```python
from build123d import *

# Parameters (mm, degrees)
SKETCH1_W                = 40.5
SKETCH1_H                = 20
BOSS_EXTRUDE1_DEPTH      = 36.1
SKETCH2_R                = 2.5
BOSS_EXTRUDE2_DEPTH      = 8
BOSS_EXTRUDE3_DEPTH      = 7.5
BOSS_EXTRUDE3_DEPTH_BACK = 48
SKETCH3_W                = 20
SKETCH3_H                = 2
SKETCH4_R                = 2
CUT_EXTRUDE1_DEPTH       = 7.5


with BuildPart() as part:
    # Sketch1 → Boss-Extrude1 (new body)
    with BuildSketch(Plane(origin=(0, 0, 0), x_dir=(1, 0, 0), z_dir=(0, 1, 0))):
        with Locations((3.506737992, 0.753901676)):
            Rectangle(SKETCH1_W, SKETCH1_H)
    extrude(amount=BOSS_EXTRUDE1_DEPTH)

    # Sketch2 → Boss-Extrude2 (add)
    with BuildSketch(Plane(origin=(0, 36.1, 0), x_dir=(1, 0, 0), z_dir=(0, 1, 0))):
        with Locations(Location((12.506737992, 0.753901676, 0), (0, 0, 270))):
            Circle(SKETCH2_R)
    extrude(amount=BOSS_EXTRUDE2_DEPTH)

    # Sketch3 → Boss-Extrude3 (add, two sides: drawn at the far end of the back side and taken through both)
    with BuildSketch(Plane.ZY.offset(16.743262008).offset(-BOSS_EXTRUDE3_DEPTH_BACK)):
        with Locations((-0.753901676, 27.6)):
            Rectangle(SKETCH3_W, SKETCH3_H)
    extrude(amount=BOSS_EXTRUDE3_DEPTH + BOSS_EXTRUDE3_DEPTH_BACK)

    # Sketch4 → Cut-Extrude1 (cut)
    with BuildSketch(Plane(origin=(0, 28.6, 0), x_dir=(1, 0, 0), z_dir=(0, 1, 0))):
        with Locations(Location((-20.493262008, 5.753901676, 0), (0, 0, 270))):
            Circle(SKETCH4_R)
        with Locations(Location((27.506737992, 5.753901676, 0), (0, 0, 270))):
            Circle(SKETCH4_R)
        with Locations(Location((-20.493262008, -4.246098324, 0), (0, 0, 270))):
            Circle(SKETCH4_R)
        with Locations(Location((27.506737992, -4.246098324, 0), (0, 0, 270))):
            Circle(SKETCH4_R)
    extrude(amount=-CUT_EXTRUDE1_DEPTH, mode=Mode.SUBTRACT)


solid = part.part
```
Geometry check sheet. Reference: the model listing, model coordinates, mm. A direction names the side the tool comes from. Coordinates: 2 decimals unless noted, no trailing zeros. Write each loop counter-clockwise with the first axis right and the second up, starting at its lowest first coordinate (ties: lowest second). Pieces come first, ordered by that corner, then holes. Notation, with made-up numbers: M 21.25,89.5 L 58.25,89.5 A20 ccw 58.25,127.5 Z; hole C -21.75,71.25 d9. An arc over 180 degrees is marked long. Use one line per item in the form item = value. Start each with the question number.
1) Section check A-A on z = 5.5. Enter the section's corners in (x, y).
2) Thickness scan on probe 1 along Y at (x, z) = (2, -4.25); probe 2 along X at (y, z) = (12.5, -8.5); probe 3 along Y at (x, z) = (24, 1.25). Record the ranges inside material, lowest first. Write a range as from..to.
3) Go/stop test with flat-tipped pins: pin 1 Ø8 at (x, z) = (-4, -4) entering from +Y; pin 2 Ø4 at (x, z) = (-21, 2) entering from -Y; pin 3 Ø3 at (x, z) = (-20.49, 4.25) entering from -Y; pin 4 Ø5 at (x, z) = (27.51, -5.75) entering from +Y. Record where each tip stops, or that it passes through.
4) Section check B-B on x = -19.5. Enter the section's corners in (y, z), and give its area (3 significant figures).
5) Release check for a two-part mould opening along Z. For faces 1 (the cylindrical face through (10.066, 40.044, -1.296)), 2 (the flat face through (28, 28.6, -1)), 3 (the cylindrical face through (27.595, 27.614, 2.248)) record: pulls with the +Z half, pulls with the -Z half, needs draft (parallel to the pull), parting line crosses it, or undercut.
6) Section check D-D on y = 15.5. Enter the section's corners in (x, z).
7) Set-up check for faces 4 (the flat face through (28, 26.6, -1)), 5 (the flat face through (-16.743, 13, -1)), 6 (the flat face through (3, 0, -1)), 7 (the flat face through (23.757, 32, -1)), 8 (the flat face through (-20, 28.6, -1)): record each of +Z, -Z, +X, -X, +Y, -Y from which the full face is reachable in a straight line by a thin tool's end or side.
8) Section check C-C on z = -9. Enter the section's corners in (x, y).
Responses:
q1.outline = M -24.24,26.6 L -22.05,26.6 L -22.05,28.6 L -24.24,28.6 Z; M -18.94,26.6 L -16.74,26.6 L -16.74,0 L 23.76,0 L 23.76,26.6 L 25.95,26.6 L 25.95,28.6 L 23.76,28.6 L 23.76,36.1 L -16.74,36.1 L -16.74,28.6 L -18.94,28.6 Z; M 29.06,26.6 L 31.26,26.6 L 31.26,28.6 L 29.06,28.6 Z
q2.probe_1 = 0..36.1
q2.probe_2 = -16.74..23.76
q2.probe_3 = 26.6..28.6
q3.pin_1 = 36.1
q3.pin_2 = 26.6
q3.pin_3 = through
q3.pin_4 = 28.6
q4.outline = M 26.6,-10.75 L 28.6,-10.75 L 28.6,-7.49 L 26.6,-7.49 Z; M 26.6,-4.02 L 28.6,-4.02 L 28.6,2.51 L 26.6,2.51 Z; M 26.6,5.98 L 28.6,5.98 L 28.6,9.25 L 26.6,9.25 Z
q4.area = 26.1 mm2
q5.face_1 = parting line crosses it
q5.face_2 = needs draft
q5.face_3 = undercut
q6.outline = M -16.74,-10.75 L 23.76,-10.75 L 23.76,9.25 L -16.74,9.25 Z
q7.face_4 = +Z, -Z, +X, -Y
q7.face_5 = +Z, -Z, -X, -Y
q7.face_6 = +Z, -Z, +X, -X, -Y
q7.face_7 = +Z, -Z, +X, +Y
q7.face_8 = +Z, -Z, -X, +Y
q8.outline = M -24.24,26.6 L -16.74,26.6 L -16.74,0 L 23.76,0 L 23.76,26.6 L 31.26,26.6 L 31.26,28.6 L 23.76,28.6 L 23.76,36.1 L -16.74,36.1 L -16.74,28.6 L -24.24,28.6 Z
